For this review, take the finished solid that the model builds, in its own axes (mm). Give positions to 0.01 mm unless a question says otherwise; leave off trailing zeros. Order: outer loops, then holes, each group sorted by start corner. A loop starts at its lowest first (then second) coordinate and runs counter-clockwise, first axis right, second up.
Item 1: Consider section A-A (z = 0.35). Give the boundary of the cut face in (x, y) (3 decimals).
Item 2: Consider section B-B (x = 130.5). Give the boundary of the cut face in (y, z), plus the area to 3 significant figures.
Item 3: For P1, Ø3, axis at x = -54, y = 20, coming from the +Z side; P2, Ø1, axis at x = -98, z = -0.5, coming from the +Y side, all flat-tipped, find the tip position at first contact; note any pin that passes through.
Item 4: For probe 1 along X at (y, z) = (19.75, -1.35) (3 decimals); probe 2 along Y at (x, z) = (-99, 1.1), list the stretches that pass through material, from the lowest coordinate up.
```python
from build123d import *

# Parameters (mm, degrees)
SKETCH1_W           = 298.45
SKETCH1_H           = 3.175
BOSS_EXTRUDE1_DEPTH = 22.225
SKETCH2_W           = 110.49
SKETCH2_H           = 3.048
SKETCH2_W_2         = 64.77
CUT_EXTRUDE1_DEPTH  = 151.904379907


with BuildPart() as part:
    # Sketch1 → Boss-Extrude1 (new body)
    with BuildSketch(Plane(origin=(0, 0, 0), x_dir=(1, 0, 0), z_dir=(0, 1, 0))):
        Rectangle(SKETCH1_W, SKETCH1_H)
    extrude(amount=BOSS_EXTRUDE1_DEPTH)

    # Sketch2 → Cut-Extrude1 (cut, through all)
    with BuildSketch(Plane.XY.offset(1.5875)):
        with Locations((-93.98, 20.701)):
            Rectangle(SKETCH2_W, SKETCH2_H)
        with Locations((93.98, 20.701)):
            Rectangle(SKETCH2_W, SKETCH2_H)
        with Locations((0, 20.701)):
            Rectangle(SKETCH2_W_2, SKETCH2_H)
    extrude(amount=-CUT_EXTRUDE1_DEPTH, mode=Mode.SUBTRACT)


solid = part.part
```
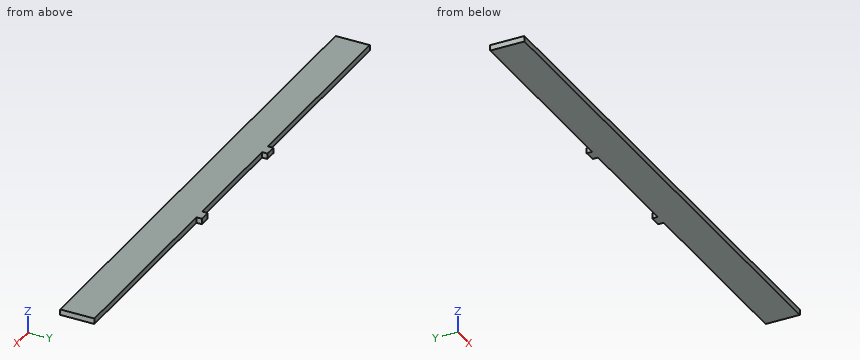
Resolved:
1. outline: (-149.225, 0) - (149.225, 0) - (149.225, 19.177) - (38.735, 19.177) - (38.735, 22.225) - (32.385, 22.225) - (32.385, 19.177) - (-32.385, 19.177) - (-32.385, 22.225) - (-38.735, 22.225) - (-38.735, 19.177) - (-149.225, 19.177) - close
2. outline: (0, -1.59) - (19.18, -1.59) - (19.18, 1.59) - (0, 1.59) - close
2. area: 60.9 mm2
3. P1: stops at z = 1.59
3. P2: stops at y = 19.18
4. probe 1: x = -38.735 to -32.385, 32.385 to 38.735
4. probe 2: y = 0 to 19.18
